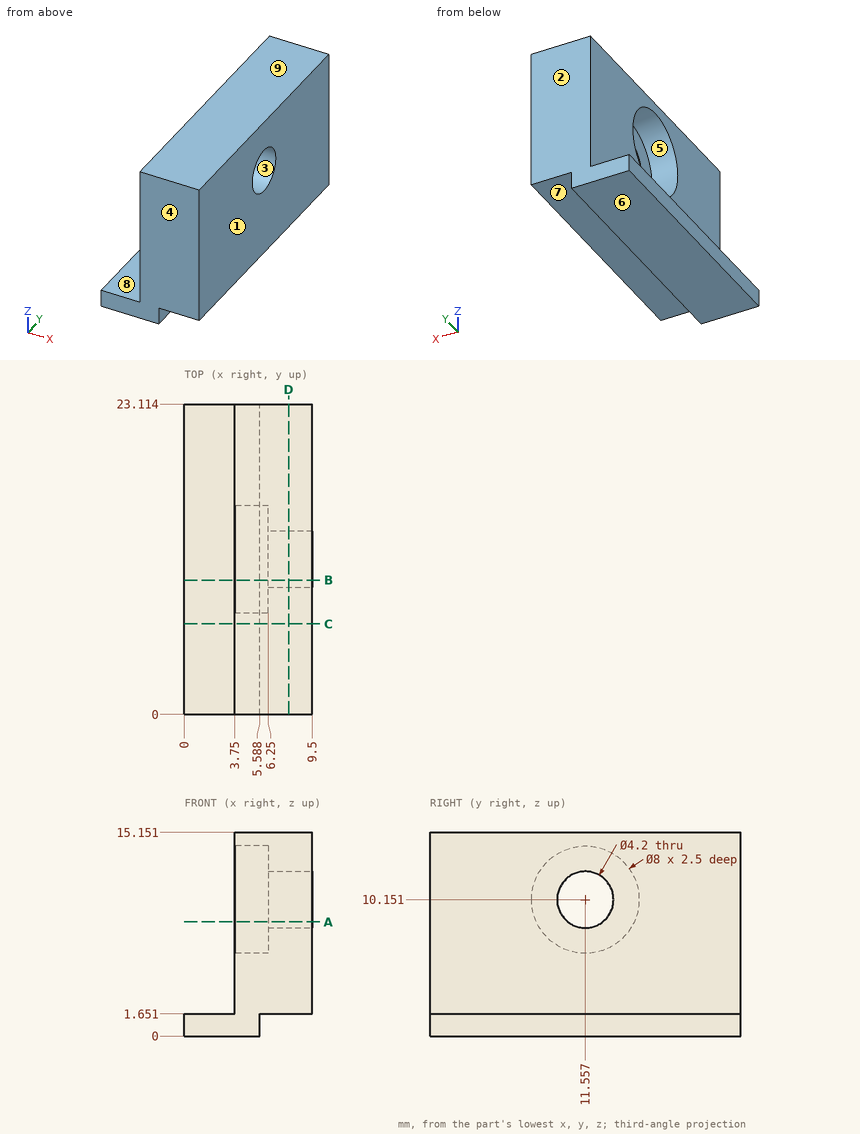
Geometry check sheet. Reference: drawing and pictorial views, mm from the part's lowest x, y, z. A direction names the side the tool comes from. Round coordinates to 2 decimals unless told otherwise and drop trailing zeros. Order: outer loops, then holes, each group sorted by start corner. A loop starts at its lowest first (then second) coordinate and runs counter-clockwise, first axis right, second up. Notation, with made-up numbers: (-16.75, 82) - (-3.75, 82) arc R22 ccw to (-3.75, 95) - close; hole circle Ø1 at (61, -5). An arc over 180 degrees is marked (long way). One line per question, with ' | ' between items. Start each with the question number.
(1) Sectioned sample at B-B on y = 10. Record the cut outline in (x, z), and give its area (3 significant figures).
(2) Sectioned sample at C-C on y = 6.75. Record the cut outline in (x, z).
(3) Depth check by flat-ended pin: pin 1 Ø3 at (x, y) = (8, 12.5) entering from -Z; pin 2 Ø8 at (y, z) = (20.5, 6.5) entering from -X; pin 3 Ø0.8 at (y, z) = (10.5, 1) entering from +X. Enter the tip coordinate at first touch or a pass-through.
(4) Access from +Z, -Z, +X, -X, +Y, -Y to the whole of each face (thin tool, end or side, straight path). Record for the marked faces 5, 6, 7, 8 and 9.
(5) Release check for a two-part mould opening along Y. For the marked faces 1, 2, 3 and 4 record: released by +Y, released by -Y, zero draft, split by the parting line, or undercut.
(6) Thickness scan on L1, parallel to Y at x = 4.75, z = 10.25; L2, parallel to X at y = 11.25, z = 12.5; L3, parallel to Y at x = 8, z = 10.25. Record the ranges inside material, lowest first. Write a range as [from, to].
(7) Sectioned sample at D-D on x = 7.75. Record the cut outline in (y, z), and give its area (3 significant figures).
(8) Sectioned sample at A-A on z = 8.5. Record the cut outline in (x, y).
Conclusion:
1) outline: (0, 0) - (5.59, 0) - (5.59, 1.65) - (9.5, 1.65) - (9.5, 8.74) - (6.25, 8.74) - (6.25, 6.47) - (3.75, 6.47) - (3.75, 1.65) - (0, 1.65) - close; (3.75, 13.84) - (6.25, 13.84) - (6.25, 11.56) - (9.5, 11.56) - (9.5, 15.15) - (3.75, 15.15) - close | area: 59.3 mm2
2) outline: (0, 0) - (5.59, 0) - (5.59, 1.65) - (9.5, 1.65) - (9.5, 15.15) - (3.75, 15.15) - (3.75, 1.65) - (0, 1.65) - close
3) pin 1: stops at z = 1.65 | pin 2: stops at x = 3.75 | pin 3: stops at x = 5.59
4) face 5: -X | face 6: -Z, +X, -X, +Y, -Y | face 7: -Z, +X, +Y, -Y | face 8: +Z, -X, +Y, -Y | face 9: +Z, +X, -X, +Y, -Y
5) face 1: zero draft | face 2: released by +Y | face 3: undercut | face 4: released by -Y
6) L1: y = [0, 7.56], [15.56, 23.11] | L2: x = [6.25, 9.5] | L3: y = [0, 9.46], [13.65, 23.11]
7) outline: (0, 1.65) - (23.11, 1.65) - (23.11, 15.15) - (0, 15.15) - close; hole circle Ø4.2 at (11.56, 10.15) | area: 298 mm2
8) outline: (3.75, 0) - (9.5, 0) - (9.5, 10.26) - (6.25, 10.26) - (6.25, 7.91) - (3.75, 7.91) - close; (3.75, 15.2) - (6.25, 15.2) - (6.25, 12.85) - (9.5, 12.85) - (9.5, 23.11) - (3.75, 23.11) - close
